Could you check a few things on this model? Use its own coordinates, in mm. Face numbers are marked on the shaded views. A direction names the side the tool comes from. Coordinates: 2 decimals unless noted, no trailing zeros. Order: outer loops, then holes, each group sorted by start corner. A loop starts at its lowest first (then second) coordinate and runs counter-clockwise, first axis right, second up. Notation, with made-up numbers: (84, 11) -> (108, 11) arc R35 cw to (108, 45) -> close; hole circle Ø6 at (66.5, -36.5). An arc over 180 degrees is marked (long way). Return JSON: item names as keys, results as strings. Group by question number.
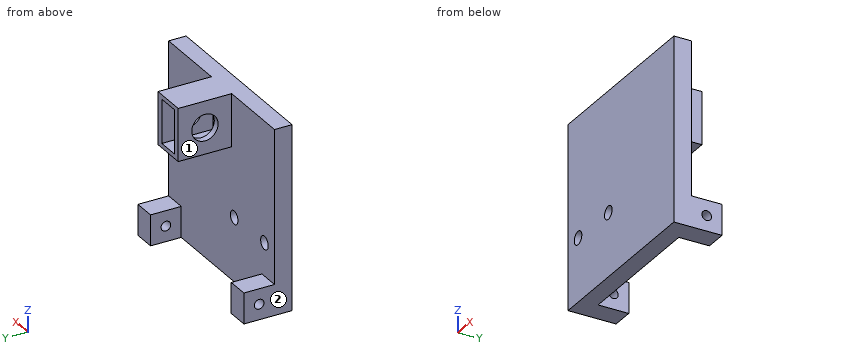
from build123d import *

# Parameters (mm, degrees)
SKETCH2_W           = 42
SKETCH2_H           = 42
BOSS_EXTRUDE1_DEPTH = 4
SKETCH4_W           = 5
SKETCH4_H           = 7
BOSS_EXTRUDE2_DEPTH = 7
SKETCH5_R           = 1.1
CUT_EXTRUDE2_DEPTH  = 5
SKETCH6_R           = 1.1
CUT_EXTRUDE3_DEPTH  = 5
SKETCH8_R           = 1.5
CUT_EXTRUDE5_DEPTH  = 4
SKETCH9_W           = 8
SKETCH9_H           = 12
BOSS_EXTRUDE3_DEPTH = 12.2
SKETCH10_W          = 5
SKETCH10_H          = 10
CUT_EXTRUDE6_DEPTH  = 11.7
SKETCH12_R          = 3
CUT_EXTRUDE7_DEPTH  = 8


with BuildPart() as part:
    # Sketch2 → Boss-Extrude1 (new body)
    with BuildSketch(Plane(origin=(0, 0, 0), x_dir=(1, 0, 0), z_dir=(0, 1, 0))):
        with Locations((-19.403711124, 0.667809886)):
            Rectangle(SKETCH2_W, SKETCH2_H)
    extrude(amount=BOSS_EXTRUDE1_DEPTH)

    # Sketch4 → Boss-Extrude2 (add)
    with BuildSketch(Plane(origin=(0, 4, 0), x_dir=(1, 0, 0), z_dir=(0, 1, 0))):
        with Locations((-37.903711124, 18.167809886)):
            Rectangle(SKETCH4_W, SKETCH4_H)
        with Locations((-0.903711124, 18.167809886)):
            Rectangle(SKETCH4_W, SKETCH4_H)
    extrude(amount=BOSS_EXTRUDE2_DEPTH)

    # Sketch5 → Cut-Extrude2 (cut)
    with BuildSketch(Plane(origin=(-35.403711124, 0, 0), x_dir=(0, 0, -1), z_dir=(1, 0, 0))):
        with Locations((18.167809886, 7.5)):
            Circle(SKETCH5_R)
    extrude(amount=-CUT_EXTRUDE2_DEPTH, mode=Mode.SUBTRACT)

    # Sketch6 → Cut-Extrude3 (cut)
    with BuildSketch(Plane.ZY.offset(3.403711124)):
        with Locations((-18.167809886, 7.5)):
            Circle(SKETCH6_R)
    extrude(amount=-CUT_EXTRUDE3_DEPTH, mode=Mode.SUBTRACT)

    # Sketch8 → Cut-Extrude5 (cut)
    with BuildSketch(Plane.XZ):
        with Locations((-36.403711124, -7.167809886)):
            Circle(SKETCH8_R)
        with Locations((-24.403711124, -7.167809886)):
            Circle(SKETCH8_R)
    extrude(amount=-CUT_EXTRUDE5_DEPTH, mode=Mode.SUBTRACT)

    # Sketch9 → Boss-Extrude3 (add)
    with BuildSketch(Plane(origin=(0, 4, 0), x_dir=(1, 0, 0), z_dir=(0, 1, 0))):
        with Locations((-19.403711124, -14.332190114)):
            Rectangle(SKETCH9_W, SKETCH9_H)
    extrude(amount=BOSS_EXTRUDE3_DEPTH)

    # Sketch10 → Cut-Extrude6 (cut)
    with BuildSketch(Plane(origin=(0, 16.2, 0), x_dir=(1, 0, 0), z_dir=(0, 1, 0))):
        with Locations((-19.403711124, -14.332190114)):
            Rectangle(SKETCH10_W, SKETCH10_H)
    extrude(amount=-CUT_EXTRUDE6_DEPTH, mode=Mode.SUBTRACT)

    # Sketch12 → Cut-Extrude7 (cut)
    with BuildSketch(Plane(origin=(-15.403711124, 0, 0), x_dir=(0, 0, -1), z_dir=(1, 0, 0))):
        with Locations((-14.332190114, 10.1)):
            Circle(SKETCH12_R)
    extrude(amount=-CUT_EXTRUDE7_DEPTH, mode=Mode.SUBTRACT)


solid = part.part
Q1. I'm going to push flat-ended pins straight in: pin 1 Ø2 at (x, y) = (-27.5, 6.5) entering from -Z; pin 2 Ø5 at (x, z) = (-24.4, -7.17) entering from +Y; pin 3 Ø1.5 at (x, z) = (-38, -20) entering from +Y; pin 4 Ø8 at (y, z) = (11, 12.5) entering from +X. Where does each tip first touch, or does it pass through?
Q2. On a 3-axis mill with a long thin cutter (end or side, diameter ignored), from which of +Z, -Z, +X, -X, +Y, -Y can I reach the whole of each face in a straight line? I mean the marked faces 1 and 2. Say none if no direction works.
Q3. I want a section at D-D on z = 1.5. Please give me the cut outline in (x, y).
Q4. I want a section at A-A on y = 10.1. Please give me the cut outline in (x, z), and give its area (3 significant figures).
Q5. I want a section at C-C on x = -24.5. Please give me the cut outline in (y, z), and give its area (3 significant figures).
Q6. I want a section at B-B on x = -19.5. Please give me the cut outline in (y, z), and give its area (3 significant figures).
Q7. I need wall thicknesses on line 1 along Z through (x, y) = (-20, 12); line 2 along X through (y, z) = (9.5, -19); line 3 along X through (y, z) = (9.5, 18.5). Which ranges of each line are inside material? Lowest first, please. Write a range as from..to.
Response values:
{
 "1": {"pin 1": "passes through", "pin 2": "stops at y = 4", "pin 3": "stops at y = 11", "pin 4": "stops at x = -15.4"},
 "2": {"face 1": "+Z, -Z, -X, +Y", "face 2": "+Z, -Z, -X, +Y, -Y"},
 "3": {"outline": "(-40.4, 0) -> (1.6, 0) -> (1.6, 4) -> (-40.4, 4) -> close"},
 "4": {"outline": "(-40.4, -21.67) -> (-35.4, -21.67) -> (-35.4, -14.67) -> (-40.4, -14.67) -> close; (-23.4, 8.33) -> (-15.4, 8.33) -> (-15.4, 11.33) -> (-16.9, 11.33) -> (-16.9, 9.33) -> (-21.9, 9.33) -> (-21.9, 11.33) -> (-23.4, 11.33) -> close; (-23.4, 17.33) -> (-21.9, 17.33) -> (-21.9, 19.33) -> (-16.9, 19.33) -> (-16.9, 17.33) -> (-15.4, 17.33) -> (-15.4, 20.33) -> (-23.4, 20.33) -> close; (-3.4, -21.67) -> (1.6, -21.67) -> (1.6, -14.67) -> (-3.4, -14.67) -> close", "area": "98.0 mm²"},
 "5": {"outline": "(0, -21.67) -> (4, -21.67) -> (4, -8.66) -> (0, -8.66) -> close; (0, -5.67) -> (4, -5.67) -> (4, 20.33) -> (0, 20.33) -> close", "area": "156 mm²"},
 "6": {"outline": "(0, -21.67) -> (4, -21.67) -> (4, 8.33) -> (16.2, 8.33) -> (16.2, 9.33) -> (4.5, 9.33) -> (4.5, 19.33) -> (16.2, 19.33) -> (16.2, 20.33) -> (0, 20.33) -> close", "area": "197 mm²"},
 "7": {"line 1": "z = 8.33..9.33, 19.33..20.33", "line 2": "x = -40.4..-35.4, -3.4..1.6", "line 3": "x = -23.4..-21.9, -16.9..-15.4"}
}
